Could you check a few things on this model? Use its own coordinates, in mm. Face numbers are marked on the shaded views. A direction names the side the tool comes from. Round coordinates to 2 decimals unless told otherwise and drop trailing zeros. Loops run counter-clockwise (first coordinate to the right, second up) from the corner with the lowest first, then second, coordinate; pieces in that order, holes last. Notation, with made-up numbers: (30.25, 88.5) -> (68.25, 88.5) arc R16 cw to (68.25, 111.5) -> close; hole circle Ø3 at (29, 10.25). An arc over 180 degrees is marked (long way). One line per item, written item: value.
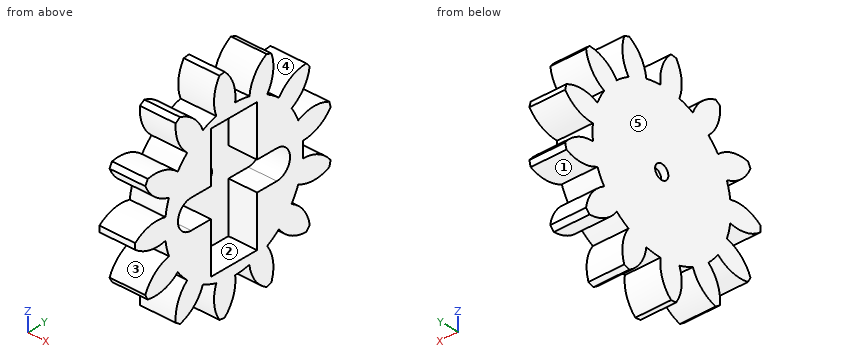
from build123d import *

# Parameters (mm, degrees)
BASPROSKE_W        = 5
BASPROSKE_H        = 15
TOOTHCUT_DEPTH     = 22.794494718
TEETHCUTS_COUNT    = 13
TEETHCUTS_ANGLE    = 332.307692308
BORSKE_R           = 1
BORE_DEPTH         = 50.0000508
CUT_EXTRUDE1_DEPTH = 4


with BuildPart() as part:
    # BasProSke → Base-Revolve (revolve)
    with BuildSketch(Plane(origin=(0, 0, 0), x_dir=(1, 0, 0), z_dir=(0, 1, 0)), mode=Mode.PRIVATE) as base_revolve_sk:
        with Locations((2.5, 7.5)):
            Rectangle(BASPROSKE_W, BASPROSKE_H)
    revolve(base_revolve_sk.sketch.rotate(Axis((-10, 0, 0), (1, 0, 0)), 180), axis=Axis((-10, 0, 0), (1, 0, 0)))

    # TooCutSke → ToothCut (cut, through all)
    with BuildSketch(Plane(origin=(0, 0, 0), x_dir=(0, 0, -1), z_dir=(1, 0, 0))):
        with BuildLine():
            ThreePointArc((1.088245291, 10.442448141), (0, 10.499), (-1.088245291, 10.442448141))
            ThreePointArc((-1.088245291, 10.442448141), (-1.646045958, 12.816546547), (-3.224884568, 14.675243258))
            ThreePointArc((-3.224884568, 14.675243258), (0, 15.0254), (3.224884568, 14.675243258))
            ThreePointArc((3.224884568, 14.675243258), (1.646045958, 12.816546547), (1.088245291, 10.442448141))
        make_face()
    toothcut = extrude(amount=TOOTHCUT_DEPTH, mode=Mode.SUBTRACT)

    # TeethCuts: ToothCut ×13 about axis
    teethcuts_axis = Axis((-10, 0, 0), (1, 0, 0))
    for i in range(1, TEETHCUTS_COUNT):
        add(toothcut.rotate(teethcuts_axis, i * TEETHCUTS_ANGLE / (TEETHCUTS_COUNT - 1)), mode=Mode.SUBTRACT)

    # BorSke → Bore (cut, symmetric)
    with BuildSketch(Plane(origin=(0, 0, 0), x_dir=(0, 0, -1), z_dir=(1, 0, 0))):
        with Locations(Location((0, 0, 0), (0, 0, 180))):
            Circle(BORSKE_R)
    extrude(amount=BORE_DEPTH, both=True, mode=Mode.SUBTRACT)

    # Sketch1 → Cut-Extrude1 (cut)
    with BuildSketch(Plane(origin=(5, 0, 0), x_dir=(0, 0, -1), z_dir=(1, 0, 0))):
        with BuildLine():
            Line((2, 6.5), (2, 3.5))
            Line((2, 3.5), (9, 3.5))
            Line((9, 3.5), (9, -3.5))
            Line((9, -3.5), (2, -3.5))
            Line((2, -3.5), (2, -6.5))
            ThreePointArc((2, -6.5), (0, -8.5), (-2, -6.5))
            Line((-2, -6.5), (-2, -3.5))
            Line((-2, -3.5), (-9, -3.5))
            Line((-9, -3.5), (-9, 3.5))
            Line((-9, 3.5), (-2, 3.5))
            Line((-2, 3.5), (-2, 6.5))
            ThreePointArc((-2, 6.5), (0, 8.5), (2, 6.5))
        make_face()
    extrude(amount=-CUT_EXTRUDE1_DEPTH, mode=Mode.SUBTRACT)


solid = part.part
(1) If we section it at A-A, the plane y = -0.5: Please give me the cut outline in (x, z), then the cut area to 3 significant figures.
Recorded:
outline: (0, -13.8) -> (5, -13.8) -> (5, -9) -> (1, -9) -> (1, -0.87) -> (0, -0.87) -> close; (0, 0.87) -> (1, 0.87) -> (1, 9) -> (5, 9) -> (5, 13.8) -> (0, 13.8) -> close
area: 64.2 mm²
(2) I'm going to push flat-ended pins straight in: pin 1 Ø1.5 at (x, y) = (2.5, -5) entering from +Z; pin 2 Ø10 at (y, z) = (9, 5.5) entering from -X; pin 3 Ø0.9 at (x, y) = (3.5, -5) entering from -Z; pin 4 Ø2 at (x, z) = (3, -5) entering from -Y. Where does each tip first touch, or does it pass through?
Recorded:
pin 1: z = 11.07
pin 2: x = 0
pin 3: z = -10.7
pin 4: y = -13.16
(3) If we section it at B-B, the plane y = -12.25: Please give me the cut outline in (x, z), then the cut area to 3 significant figures.
Recorded:
outline: (0, -7.43) -> (5, -7.43) -> (5, -4.85) -> (0, -4.85) -> close; (0, -1.57) -> (5, -1.57) -> (5, 1.57) -> (0, 1.57) -> close; (0, 4.85) -> (5, 4.85) -> (5, 7.43) -> (0, 7.43) -> close
area: 41.6 mm²
(4) For the marked faces 1, 2 and 3, which set-ups out of +Z, -Z, +X, -X, +Y, -Y let a thin tool reach every point of the face, with its end or its side?
Recorded:
face 1: +X, -X
face 2: +X
face 3: +X, -X, -Y
(5) Thinking about a two-plate mould opening in Y: for the marked faces 4 and 5, which applies, released by +Y, released by -Y, zero draft, split by the parting line, or undercut?
Recorded:
face 4: undercut
face 5: zero draft
(6) If I drill on L1, parallel to Y at x = 0.2, z = 0; L2, parallel to Y at x = 0.4, z = 12.25; L3, parallel to Z at x = 4.2, y = -12.25, over which ranges is the centre line in solid material (lowest first)?
Recorded:
L1: -15 to -1, 1 to 10.5
L2: -8.66 to -7.34, -3.03 to 0.1, 3.01 to 5.97
L3: -7.43 to -4.85, -1.57 to 1.57, 4.85 to 7.43
